Autodesk Inventor part; units mm, degrees
ref_plane "Work Plane4" through (0, 0, 9.525) normal (0, 0, 1) x (1, 0, 0)
ref_plane "Work Plane3" through (0, 0, 9.525) normal (0, 0, 1) x (1, 0, 0)
ref_plane "YZ Plane" through (0, 0, 0) normal (1, 0, 0) x (0, 1, 0)
sketch "Sketch1" plane through (0, 0, 0) normal (0, 0, 1) x (1, 0, 0)
  line L0 (0, 0) -> (6.35, 0)
  line L1 (6.35, 0) -> (6.35, 12.7)
  line L2 (6.35, 12.7) -> (25.4, 12.7)
  line L3 (25.4, 12.7) -> (25.4, 0)
  line L4 (25.4, 0) -> (31.75, 0)
  circle A0 centre (15.875, 25.4) radius 4.7815
  line L5 (-323.85, 246.5917) -> (-305.435, 246.5917)
  line L6 (-323.85, 142.875) -> (-83.185, 142.875)
  line L7 (-83.185, 142.875) -> (-37.2427, 114.1611)
  line L8 (-32.385, 142.875) -> (22.225, 142.875)
  line L9 (-32.385, 116.8535) -> (-32.385, 142.875)
  arc A1 (-37.2427, 114.1611) -> (-32.385, 116.8535) centre (-35.56, 116.8535) ccw
  line L10 (-323.85, 168.275) -> (-323.85, 246.5917)
  line L11 (-323.85, 246.5917) -> (-304.8, 246.5917)
  line L12 (-323.85, 168.275) -> (-323.85, 142.875)
  line L13 (0, 0) -> (0, 38.1)
  line L14 (53.975, -21.4734) -> (53.975, 330.2514) construction
  line L15 (0, 38.1) -> (22.225, 63.5)
  line L16 (22.225, 63.5) -> (22.225, 142.875)
  line L17 (53.975, 63.5) -> (53.975, 168.275)
  line L18 (53.975, 63.5) -> (53.975, 168.275)
  line L19 (22.225, 63.5) -> (22.225, 142.875)
  line L20 (-32.385, 142.875) -> (22.225, 142.875)
  line L21 (-83.185, 142.875) -> (-323.85, 142.875)
  line L22 (31.75, 0) -> (38.1, 0)
  line L23 (38.1, 0) -> (38.1, 38.1)
  line L24 (38.1, 38.1) -> (53.975, 63.5)
  line L25 (38.1, 0) -> (31.75, 0)
  line L26 (-304.8, 246.5917) -> (-213.7569, 168.275)
  line L27 (-233.2314, 168.275) -> (-302.26, 227.6544)
  line L28 (53.975, 168.275) -> (-213.7569, 168.275)
  line L29 (-233.2314, 168.275) -> (-302.26, 168.275)
  line L30 (-302.26, 168.275) -> (-233.2314, 168.275)
  line L31 (-213.7569, 168.275) -> (53.975, 168.275)
  circle A2 centre (-285.75, 149.225) radius 1.5875
  circle A3 centre (-285.75, 161.925) radius 1.5875
  line L32 (-302.26, 168.275) -> (-302.26, 227.6544)
  point P0 (-32.385, 111.125)
  point P1 (-359.41, 168.275)
  dimension "d0" = 6.35
  dimension "d1" = 12.7
  dimension "d2" = 19.05
  dimension "d3" = 6.35
  dimension "d4" = 12.7
  dimension "d5" = 9.5631
  dimension "d6" = 12.7
  dimension "d8" = 377.825
  dimension "d17" = 103.7167
  dimension "d19" = 9.525
  dimension "d25" = 31.75
  dimension "d26" = 3.175
  dimension "d27" = 50.8
  dimension "d30" = 19.05
  dimension "d63" = 38.1
  dimension "d68" = 0
  dimension "d69" = 54.61
  dimension "d71" = 22.225
  dimension "d72" = 0
  dimension "d74" = 79.375
  dimension "d76" = 240.665
  dimension "d87" = 6.35
  dimension "d88" = 38.1
  dimension "d89" = 25.4
  dimension "d91" = 25.4
  dimension "d94" = 12.7
  dimension "d97" = 40.703
  dimension "d98" = 267.7319
  dimension "d109" = 3.175
  dimension "d110" = 3.175
  dimension "d111" = 38.1
  dimension "d112" = 38.1
  dimension "d113" = 6.35
  dimension "d114" = 6.35
  dimension "d135" = 25.4
  dimension "d136" = 25.4
  dimension "d143" = 21.59
ref_plane "Work Plane4" through (0, 0, 9.525) normal (0, 0, 1) x (1, 0, 0)
ref_plane "Work Plane3" through (0, 0, 9.525) normal (0, 0, 1) x (1, 0, 0)
extrude "Extrusion9" add sketch "Sketch1" along normal blind 6.35 contours L13 L15 L16 L8 L9 A1 L7 L6 L12 L10 L5 L11 L26 L28 L17 L24 L23 L22 L4 L3 L2 L1 L0 | A2 | A3
sketch "Sketch8" plane through (0, 0, 6.35) normal (0, 0, 1) x (1, 0, 0)
  line L0 (-304.8, 246.5917) -> (-323.85, 246.5917)
  line L1 (-323.85, 246.5917) -> (-323.85, 142.875)
  circle A0 centre (-309.105, 218.3215) radius 1.905
  circle A1 centre (-319.405, 196.6215) radius 1.905
  line L2 (-32.385, 142.875) -> (22.225, 142.875)
  line L3 (22.225, 142.875) -> (22.225, 63.5)
  circle A2 centre (36.97, 101.6) radius 1.905
  circle A3 centre (26.67, 79.9) radius 1.905
  dimension "d101" = 3.81
  dimension "d102" = 3.81
  dimension "d104" = 28.2702
  dimension "d105" = 4.445
  dimension "d147" = 21.7
  dimension "d148" = 10.3
  dimension "d149" = 3.81
  dimension "d150" = 3.81
  dimension "d151" = 21.7
  dimension "d152" = 10.3
  dimension "d153" = 41.275
  dimension "d154" = 4.445
extrude "Extrusion10" cut sketch "Sketch8" against normal blind 6.35
sketch "Sketch9" plane through (0, 0, 6.35) normal (0, 0, 1) x (1, 0, 0)
  line L0 (-323.85, 246.5917) -> (-323.85, 142.875)
  line L1 (-323.85, 142.875) -> (-83.185, 142.875)
  circle A0 centre (-285.75, 155.575) radius 1.5875
  circle A1 centre (-285.75, 147.6375) radius 1.5875
  dimension "d115" = 3.175
  dimension "d116" = 3.175
  dimension "d117" = 38.1
  dimension "d118" = 38.1
  dimension "d119" = 4.7625
  dimension "d124" = 7.9375
extrude "Extrusion11" cut sketch "Sketch9" against normal blind 6.35
fillet "Fillet8" radius 3.175 14 edges at (-304.8, 246.5917, 3.175) (-323.85, 246.5917, 3.175) (-213.7569, 168.275, 3.175) (53.975, 168.275, 3.175) (53.975, 63.5, 3.175) (38.1, 38.1, 3.175) (0, 0, 3.175) (0, 38.1, 3.175) (22.225, 142.875, 3.175) (22.225, 63.5, 3.175) (-83.185, 142.875, 3.175) (-32.385, 142.875, 3.175) (-323.85, 142.875, 3.175) (-302.26, 227.6544, 3.175)
fillet "Fillet9" radius 3.175 1 edges at (38.1, 0, 3.175)
sketch "Sketch11" plane through (0, 0, 6.35) normal (0, 0, 1) x (1, 0, 0)
  line L0 (53.975, 64.4106) -> (53.975, 165.1)
  arc A0 (53.975, 165.1) -> (50.8, 168.275) centre (50.8, 165.1) ccw
  line L1 (50.8, 168.275) -> (-212.5792, 168.275)
  arc A1 (-214.6497, 169.043) -> (-212.5792, 168.275) centre (-212.5792, 171.45) ccw
  line L2 (-233.2314, 168.275) -> (-302.26, 168.275)
  line L3 (-297.0145, 223.1421) -> (-233.2314, 168.275)
  line L4 (-302.26, 161.925) -> (-233.2314, 161.925)
  line L5 (-233.2314, 168.275) -> (-225.8496, 161.925)
  line L6 (-225.8496, 161.925) -> (-233.2314, 161.925)
  line L7 (-214.6497, 169.043) -> (-206.375, 161.925)
  line L8 (-206.375, 161.925) -> (53.975, 161.925)
  line L9 (-302.26, 168.275) -> (-302.26, 161.925)
  point P0 (0, 0)
  dimension "d139" = 6.35
  dimension "d144" = 6.35
extrude "Extrusion13" cut sketch "Sketch11" against normal blind 25.4
fillet "Fillet11" radius 3.175 2 edges at (-302.26, 161.925, 3.175) (-225.8496, 161.925, 3.175)
properties part number "Rebuild Left Climber Hook" material "Aluminum 6061"
CAD build for the part. Positions are in the model's coordinates, mm. A direction names the side the tool comes from. Coordinates: 2 decimals unless noted, no trailing zeros. Write each loop counter-clockwise with the first axis right and the second up, starting at its lowest first coordinate (ties: lowest second). Pieces come first, ordered by that corner, then holes. Notation, with made-up numbers: (1.25, 42) -> (31.25, 42) arc R12 cw to (31.25, 47) -> close; hole circle Ø11 at (45.25, 43.5). An arc over 180 degrees is marked (long way). Use CSV: the item, a comma, the result in double quotes. Start each with the question number.
Item 1: Band-saw the part on A-A, the plane y = 25.4. Write the cut outline in (x, z), plus the area to 3 significant figures.
Item 2: Wall check: probe 1 along Y at (x, z) = (26.67, 3) (3 decimals); probe 2 along Y at (x, z) = (36.97, 5) (3 decimals); probe 3 along X at (y, z) = (79.9, 4.75) (3 decimals). Give the ranges that are in metal, low to high.
Item 3: Band-saw the part on D-D, the plane x = -183.5. Write the cut outline in (y, z) (3 decimals), plus the area to 3 significant figures.
Item 4: Band-saw the part on C-C, the plane z = 1.25. Give the number of separate pieces and of enclosed holes in the cut face, plus the area to 3 significant figures.
Item 5: Tool access for faces 1 (the flat face through (10.968, 50.635, 3.131)), 2 (the flat face through (-122, 151, 0)): list every direction of +Z, -Z, +X, -X, +Y, -Y with a clear straight run to the whole face (end or side of a thin tool).
Item 6: Two-plate mould, pull along X, no slides. Class faces 3 (the cylindrical face through (18.081, 29.642, 3.131)), 4 (the flat face through (45.93, 50.63, 3.13)), 5 (the flat face through (-122, 151, 6.35)): +X half, -X half, draft (parallel to the pull), parting line (faces both ways), or undercut.
Item 7: Band-saw the part on B-B, the plane x = -272.5. Write the cut outline in (y, z) (3 decimals).
Item 8: Drop flat-ended pins along their axis: P1, Ø3, axis at y = 9, z = 3, coming from the -X side; P2, Ø3, axis at y = 183, z = 4, coming from the +X side; P3, Ø1.9, axis at y = 4, z = 4.5, coming from the +X side. Give the stop position or say it passes through.
Response values:
1,outline,"(0, 0) -> (11.09, 0) -> (11.09, 6.35) -> (0, 6.35) -> close; (20.66, 0) -> (38.1, 0) -> (38.1, 6.35) -> (20.66, 6.35) -> close"
1,area,"181 mm2"
2,probe 1,"y = 0 to 77.995, 81.805 to 161.925"
2,probe 2,"y = 0.746 to 99.695, 103.505 to 161.925"
2,probe 3,"x = 22.225 to 24.765, 28.575 to 53.975"
3,outline,"(142.875, 0) -> (161.925, 0) -> (161.925, 6.35) -> (142.875, 6.35) -> close"
3,area,"121 mm2"
4,separate pieces,"1"
4,enclosed holes,"8"
4,area,"15,800 mm2"
5,face 1,"+Z, -Z, -X"
5,face 2,"-Z, +X, -X, +Y, -Y"
6,face 3,"undercut"
6,face 4,"+X half"
6,face 5,"draft"
7,outline,"(142.875, 0) -> (161.925, 0) -> (161.925, 6.35) -> (142.875, 6.35) -> close; (202.054, 0) -> (218.807, 0) -> (218.807, 6.35) -> (202.054, 6.35) -> close"
8,P1,"stops at x = 0"
8,P2,"stops at x = -229.13"
8,P3,"stops at x = 38.1"
